from build123d import *

# Parameters (mm, degrees)
SKETCH2_R               = 12.5
BOSS_EXTRUDE1_DEPTH     = 6
SKETCH3_R               = 6.5
SKETCH3_R_2             = 2.5
BOSS_EXTRUDE2_DEPTH     = 7
SKETCH4_R               = 1.2
CUT_EXTRUDE1_DEPTH      = 25
CUT_EXTRUDE1_DEPTH_BACK = 25
SKETCH5_R               = 1.2
CUT_EXTRUDE2_DEPTH      = 25
CIRPATTERN1_COUNT       = 6


with BuildPart() as part:
    # Sketch2 → Boss-Extrude1 (new body)
    with BuildSketch(Plane.XY):
        Circle(SKETCH2_R)
    extrude(amount=BOSS_EXTRUDE1_DEPTH)

    # Sketch3 → Boss-Extrude2 (add)
    with BuildSketch(Plane.XY.offset(6)):
        Circle(SKETCH3_R)
        Circle(SKETCH3_R_2, mode=Mode.SUBTRACT)
    extrude(amount=BOSS_EXTRUDE2_DEPTH)

    # Sketch4 → Cut-Extrude1 (cut, two sides)
    with BuildSketch(Plane(origin=(0, 0, 0), x_dir=(1, 0, 0), z_dir=(0, 1, 0))) as cut_extrude1_sk:
        with Locations((0, -9.5)):
            Circle(SKETCH4_R)
    extrude(amount=CUT_EXTRUDE1_DEPTH, mode=Mode.SUBTRACT)
    extrude(cut_extrude1_sk.sketch, amount=-CUT_EXTRUDE1_DEPTH_BACK, mode=Mode.SUBTRACT)

    # Sketch5 → Cut-Extrude2 (cut, symmetric)
    with BuildSketch(Plane.XY.offset(6)):
        with Locations((0, 9.5)):
            Circle(SKETCH5_R)
    cut_extrude2 = extrude(amount=CUT_EXTRUDE2_DEPTH, both=True, mode=Mode.SUBTRACT)

    # CirPattern1: Cut-Extrude2 ×6 about axis
    cirpattern1_axis = Axis((0, 0, 0), (0, 0, 1))
    for i in range(1, CIRPATTERN1_COUNT):
        add(cut_extrude2.rotate(cirpattern1_axis, i * 360 / CIRPATTERN1_COUNT), mode=Mode.SUBTRACT)


solid = part.part
The listing builds one solid part. Answer for the finished solid, in the listing's coordinates (mm). A direction names the side the tool comes from. Coordinates: 2 decimals unless noted, no trailing zeros. Order: outer loops, then holes, each group sorted by start corner. A loop starts at its lowest first (then second) coordinate and runs counter-clockwise, first axis right, second up. Notation, with made-up numbers: (64, 9) -> (120, 9) arc R19 cw to (120, 26) -> close; hole circle Ø10 at (68.25, 32). An arc over 180 degrees is marked (long way). Answer in a Markdown table with one row per item. Add a question column.
Item 1: Which of the six approach directions +Z, -Z, +X, -X, +Y, -Y give full straight-line access (tool end or side, diameter ignored) to faces 1 (the face through (5, -5, 6)), 2 (the face through (-7.083, -4.39, 3.042))?
Item 2: Determine the mould class of faces 3 (the face through (-0.26, 8.33, 3.04)), 4 (the face through (-1.409, -6.345, 9.451)), 5 (the face through (3, 0, 13)) for opening direction X: +X half, -X half, draft (parallel to the pull), parting line (faces both ways), or undercut.
Item 3: Find the intervals of material crossed by L1, parallel to Y at x = 0, z = 3.15; L2, parallel to Z at x = 0, y = -3.6; L3, parallel to X at y = -5.75, z = 5, in increasing order. Write a range as from..to.
Item 4: Each of these flat-tipped pins is pushed along its axis until it touches: P1, Ø1.5, axis at x = -3.5, z = 3.5, coming from the -Y side; P2, Ø1, axis at y = -5, z = 6, coming from the -X side; P3, Ø3, axis at x = 0, y = -9.5, coming from the +Z side. Where does it stop, or does it pass through?
Item 5: Find section A-A (x = 0). Write down the section's boundary in (y, z), then the cut area to 3 significant figures.
Item 6: Find section C-C (z = 9.5). Write down the section's boundary in (x, y), then the cut area to 3 significant figures.
Item 7: Find section B-B (y = 0). Write down the section's boundary in (x, z), then the cut area to 3 significant figures.
Item 8: Find section D-D (y = 10). Write down the section's boundary in (x, z).
Result set:
| question | item | result |
|---|---|---|
| 1 | face 1 | +Z |
| 1 | face 2 | +Z, -Z |
| 2 | face 3 | undercut |
| 2 | face 4 | parting line |
| 2 | face 5 | draft |
| 3 | L1 | y = -12.5..-10.7, -8.3..8.3, 10.7..12.5 |
| 3 | L2 | z = 0..8.3, 10.7..13 |
| 3 | L3 | x = -11.1..-8.89, -7.56..7.56, 8.89..11.1 |
| 4 | P1 | stops at y = -12.19 |
| 4 | P2 | stops at x = -11.66 |
| 4 | P3 | stops at z = 6 |
| 5 | outline | (-12.5, 0) -> (-10.7, 0) -> (-10.7, 6) -> (-12.5, 6) -> close; (-8.3, 0) -> (8.3, 0) -> (8.3, 6) -> (6.5, 6) -> (6.5, 8.3) -> (2.5, 8.3) -> (2.5, 6) -> (-2.5, 6) -> (-2.5, 8.3) -> (-6.5, 8.3) -> (-6.5, 6) -> (-8.3, 6) -> close; (-6.5, 10.7) -> (-2.5, 10.7) -> (-2.5, 13) -> (-6.5, 13) -> close; (2.5, 10.7) -> (6.5, 10.7) -> (6.5, 13) -> (2.5, 13) -> close; (10.7, 0) -> (12.5, 0) -> (12.5, 6) -> (10.7, 6) -> close |
| 5 | area | 158 mm² |
| 6 | outline | (-1.2, -6.39) -> (-1.2, -2.19) arc R2.5 cw to (-1.2, 2.19) -> (-1.2, 6.39) arc R6.5 ccw to start; (1.2, -6.39) arc R6.5 ccw to (1.2, 6.39) -> (1.2, 2.19) arc R2.5 cw to (1.2, -2.19) -> close |
| 6 | area | 93.6 mm² |
| 7 | outline | (-12.5, 0) -> (12.5, 0) -> (12.5, 6) -> (6.5, 6) -> (6.5, 13) -> (2.5, 13) -> (2.5, 6) -> (-2.5, 6) -> (-2.5, 13) -> (-6.5, 13) -> (-6.5, 6) -> (-12.5, 6) -> close |
| 7 | area | 206 mm² |
| 8 | outline | (-7.5, 0) -> (-1.09, 0) -> (-1.09, 6) -> (-7.5, 6) -> close; (1.09, 0) -> (7.5, 0) -> (7.5, 6) -> (1.09, 6) -> close |
